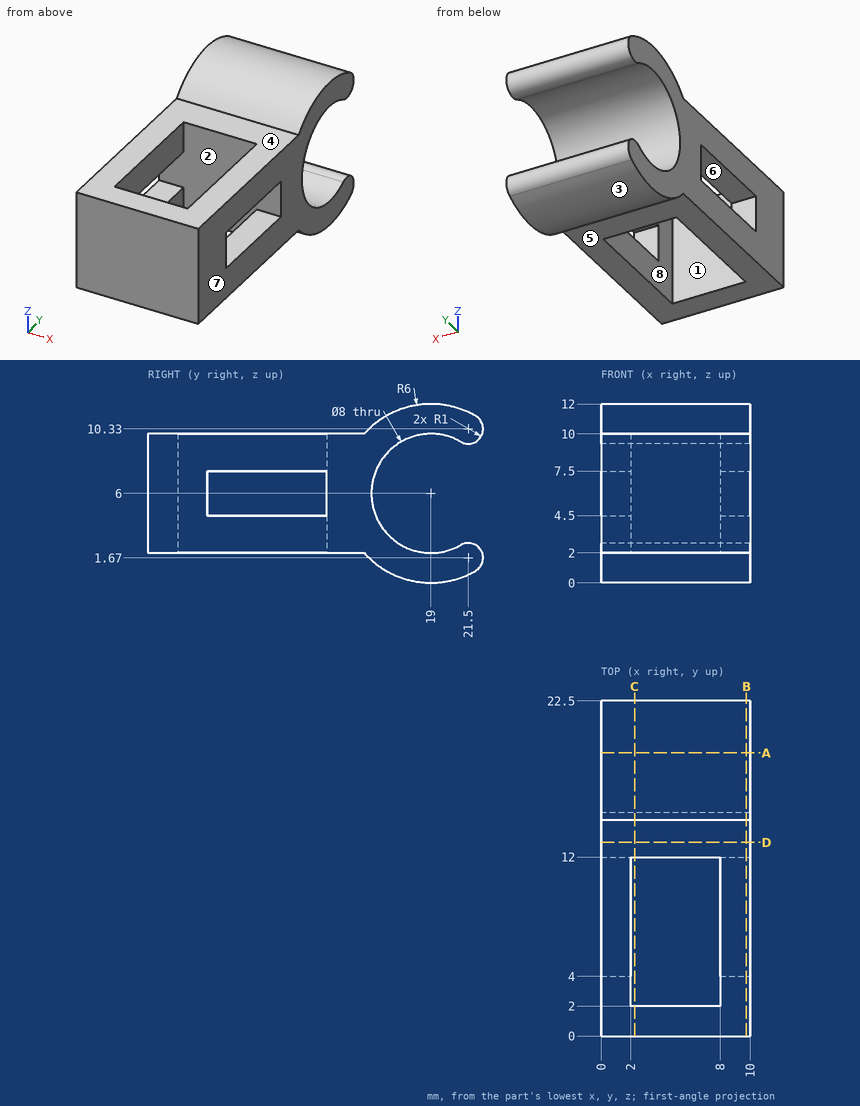
Here's the drawing with two shaded views (mm, measured from the low corner). I have some questions. A direction names the side the tool comes from. Coordinates: 2 decimals unless noted, no trailing zeros. Order: outer loops, then holes, each group sorted by start corner. A loop starts at its lowest first (then second) coordinate and runs counter-clockwise, first axis right, second up. Notation, with made-up numbers: (19, 35) -> (36, 35) arc R26 ccw to (36, 62) -> close; hole circle Ø1 at (61, 80.25). An arc over 180 degrees is marked (long way). Write each question's results on one line, items separated by ' | '.
Item 1: I want a section at C-C, the plane x = 2.25. Write out the boundary of the cut face in (y, z), then the cut area to 3 significant figures.
Results are:
outline: (0, 2) -> (2, 2) -> (2, 10) -> (0, 10) -> close; (12, 2) -> (14.53, 2) arc R6 ccw to (22, 0.8) arc R1 ccw to (21, 2.54) arc R4 cw (long way) to (21, 9.46) arc R1 ccw to (22, 11.2) arc R6 ccw to (14.53, 10) -> (12, 10) -> close | area: 72.9 mm²
Item 2: I want a section at A-A, the plane y = 19. Write out the boundary of the cut face in (x, z).
Results are:
outline: (0, 0) -> (10, 0) -> (10, 2) -> (0, 2) -> close; (0, 10) -> (10, 10) -> (10, 12) -> (0, 12) -> close
Item 3: I'm going to push flat-ended pins straight in: pin 1 Ø1.5 at (x, y) = (4.5, 15.5) entering from +Z; pin 2 Ø6 at (x, z) = (3, 4.5) entering from +Y; pin 3 Ø0.6 at (x, z) = (1.5, 6.5) entering from +Y; pin 4 Ø2 at (x, z) = (8.5, 6.5) entering from +Y. Where does each tip first touch, or does it pass through?
Results are:
pin 1: z = 11.33 | pin 2: y = 22.5 | pin 3: y = 15.08 | pin 4: y = 15.29
Item 4: If I drill on line 1 along Z through (x, y) = (2.25, 19); line 2 along X through (y, z) = (2.25, 9.5); line 3 along Y through (x, z) = (1, 9.5), over which ranges is the centre line in solid material (lowest first)?
Results are:
line 1: 0 to 2, 10 to 12 | line 2: 0 to 2, 8 to 10 | line 3: 0 to 17.06, 20.94 to 22.06
Item 5: I want a section at B-B, the plane x = 9.75. Write out the boundary of the cut face in (y, z), then the cut area to 3 significant figures.
Results are:
outline: (0, 2) -> (14.53, 2) arc R6 ccw to (22, 0.8) arc R1 ccw to (21, 2.54) arc R4 cw (long way) to (21, 9.46) arc R1 ccw to (22, 11.2) arc R6 ccw to (14.53, 10) -> (0, 10) -> close; hole (4, 4.5) -> (12, 4.5) -> (12, 7.5) -> (4, 7.5) -> close | area: 129 mm²
Item 6: Which directions (+Z, -Z, +X, -X, +Y, -Y) give clear straight access to the entire face, cutting with the end or side of a thin tool? Please do the marked faces 4, 5, 6, 7 and 8.
Results are:
face 4: +Z, +X, -X, -Y | face 5: -Z, +X, -X, -Y | face 6: +X, -X | face 7: +Z, -Z, +X, +Y, -Y | face 8: +Z, -Z
Item 7: If we mould it in two halves opening along Z, with no side actions, what happens to the marked faces 1, 2 and 3? For each: +Z half, -Z half, draft (parallel to the pull), parting line (faces both ways), or undercut.
Results are:
face 1: draft | face 2: undercut | face 3: -Z half
Item 8: I want a section at D-D, the plane y = 13. Write out the boundary of the cut face in (x, z), then the cut area to 3 significant figures.
Results are:
outline: (0, 2) -> (10, 2) -> (10, 10) -> (0, 10) -> close | area: 80.0 mm²
